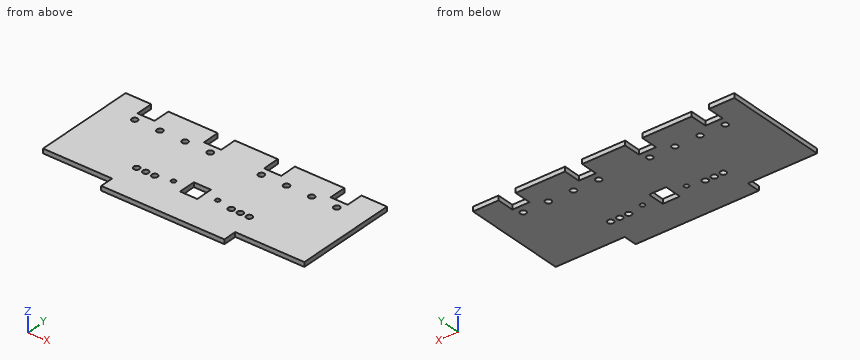
```python
from build123d import *

# Parameters (mm, degrees)
SKETCH_R      = 2
PAD_DEPTH     = 3
SKETCH001_R   = 1.5
SKETCH001_W   = 3
SKETCH001_H   = 90.076996
SKETCH001_H_2 = 90.92247
SKETCH001_W_2 = 11.4
SKETCH001_H_3 = 11.4
POCKET_DEPTH  = 3.001


with BuildPart() as part:
    # Sketch → Pad (new body)
    with BuildSketch(Plane.XY):
        Polygon((0, 77.4), (20, 77.4), (20, 66), (31.4, 66), (31.4, 77.4), (64.3, 77.4), (64.3, 66), (75.7, 66), (75.7, 77.4), (90, 77.4), (90, 0), (49, 0), (49, 9), (0, 9), align=None)
        with Locations((52.5, 25)):
            Circle(SKETCH_R, mode=Mode.SUBTRACT)
        with Locations((58.5, 25)):
            Circle(SKETCH_R, mode=Mode.SUBTRACT)
        with Locations((64.5, 25)):
            Circle(SKETCH_R, mode=Mode.SUBTRACT)
        with Locations((22.74, 60.4)):
            Circle(SKETCH_R, mode=Mode.SUBTRACT)
        with Locations((39.48, 60.4)):
            Circle(SKETCH_R, mode=Mode.SUBTRACT)
        with Locations((56.22, 60.4)):
            Circle(SKETCH_R, mode=Mode.SUBTRACT)
        with Locations((72.96, 60.4)):
            Circle(SKETCH_R, mode=Mode.SUBTRACT)
    pad = extrude(amount=PAD_DEPTH)

    # Mirrored: Pad across face of Pad
    add(pad.mirror(Plane(origin=(90, 38.7, 1.5), x_dir=(0, 1, 0), z_dir=(1, 0, 0))))

    # Sketch001 → Pocket (cut, through all)
    with BuildSketch(Plane.XY.offset(3)):
        with Locations((104.7, 27.1)):
            Circle(SKETCH001_R)
        with Locations((75.3, 27.1)):
            Circle(SKETCH001_R)
        with Locations((1.5, 45.038498)):
            Rectangle(SKETCH001_W, SKETCH001_H)
        with Locations((178.5, 45.461235)):
            Rectangle(SKETCH001_W, SKETCH001_H_2)
        with Locations((90, 27.1)):
            Rectangle(SKETCH001_W_2, SKETCH001_H_3)
    extrude(amount=-POCKET_DEPTH, mode=Mode.SUBTRACT)


solid = part.part
```
The model under review builds one solid part; all positions refer to its coordinate system, in mm. Round coordinates to 2 decimals unless told otherwise and drop trailing zeros. Order: outer loops, then holes, each group sorted by start corner. A loop starts at its lowest first (then second) coordinate and runs counter-clockwise, first axis right, second up. Notation, with made-up numbers: (30, -14.5) - (61, -14.5) arc R15 cw to (61, -9.5) - close; hole circle Ø7 at (62.5, -15). An arc over 180 degrees is marked (long way). Answer in a Markdown table with one row per item.
(1) Take a section at A-A on x = 127.5. Write out the cut boundary in (y, z), plus the area to 3 significant figures.
Result set:
| item | result |
|---|---|
| outline | (0, 0) - (23, 0) - (23, 3) - (0, 3) - close; (27, 0) - (77.4, 0) - (77.4, 3) - (27, 3) - close |
| area | 220 mm2 |
(2) Clearance check with flat-ended pins moving along their axes: P1, Ø1, axis at x = 89.5, z = 0.5, coming from the -Y side; P2, Ø1.5, axis at x = 18.5, z = 2, coming from the -Y side; P3, Ø1.5, axis at x = 70.5, z = 2, coming from the +Y side. State where each tip first meets the part, or that it passes through.
Result set:
| item | result |
|---|---|
| P1 | stops at y = 0 |
| P2 | stops at y = 9 |
| P3 | stops at y = 66 |
(3) For line 1 (X direction, y = 67, z = 0.4); line 2 (Y direction, x = 56.22, z = 1.8); line 3 (Y direction, x = 107.04, z = 1.35), list the stretches that pass through material, from the lowest coordinate up. Write a range as from..to.
Result set:
| item | result |
|---|---|
| line 1 | x = 3..20, 31.4..64.3, 75.7..104.3, 115.7..148.6, 160..177 |
| line 2 | y = 0..58.4, 62.4..77.4 |
| line 3 | y = 0..58.4, 62.4..66 |
(4) Take a section at D-D on x = 44. Write out the cut boundary in (y, z).
Result set:
| item | result |
|---|---|
| outline | (9, 0) - (77.4, 0) - (77.4, 3) - (9, 3) - close |
(5) Take a section at B-B on y = 60.4. Count the separate pieces of the cut face and the enclosed holes in it, plus the area to 3 significant figures.
Result set:
| item | result |
|---|---|
| separate pieces | 9 |
| enclosed holes | 0 |
| area | 426 mm2 |
